For this review, take the finished solid that the model builds, in its own axes (mm). Face numbers are marked on the shaded views. A direction names the side the tool comes from. Give positions to 0.01 mm unless a question says otherwise; leave off trailing zeros. Write each loop counter-clockwise with the first axis right and the second up, starting at its lowest first coordinate (ties: lowest second). Pieces come first, ordered by that corner, then holes. Notation, with made-up numbers: M 73.25,29.25 L 80.25,29.25 A5 ccw 80.25,38.25 Z; hole C 77,60 d8. An arc over 180 degrees is marked long. Write item = value, one per line.
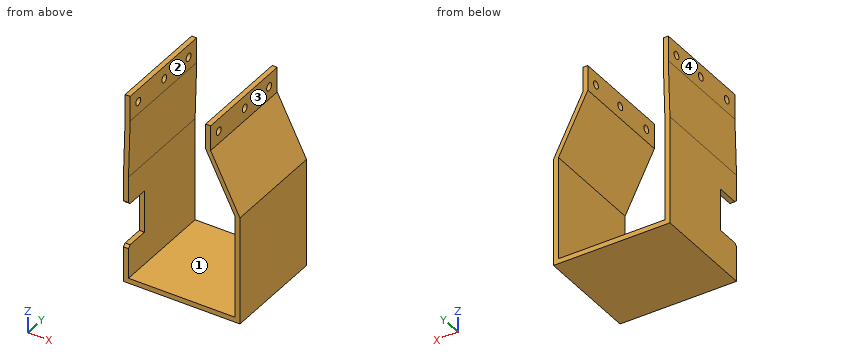
Autodesk Inventor part; units mm, degrees
ref_plane "YZ Plane" through (0, 0, 0) normal (1, 0, 0) x (0, 1, 0)
ref_plane "XZ Plane" through (0, 0, 0) normal (0, 1, 0) x (-1, 0, 0)
ref_plane "XY Plane" through (0, 0, 0) normal (0, 0, 1) x (1, 0, 0)
sketch "Sketch3" plane through (0, 0, 0) normal (0, 1, 0) x (-1, 0, 0)
  line L0 (0, 0) -> (15, 0) construction
  line L1 (0, 0) -> (-15, 0) construction
  line L2 (15, 0) -> (15, -10)
  line L3 (15, -10) -> (17, -10)
  line L4 (17, -10) -> (17, 0)
  line L5 (17, 0) -> (15, 0)
  line L6 (-15, 0) -> (-15, -10)
  line L7 (-15, -10) -> (-17, -10)
  line L8 (-17, -10) -> (-17, 0)
  line L9 (-17, 0) -> (-15, 0)
  line L10 (0, 0) -> (0, -74) construction
  line L11 (0, -74) -> (15.65, -74)
  line L12 (0, -74) -> (-26.65, -74)
  line L13 (15.65, -74) -> (15.65, -76)
  line L14 (15.65, -76) -> (-26.65, -76)
  line L15 (-26.65, -76) -> (-26.65, -74)
  line L16 (15.65, -76) -> (17.65, -76)
  line L17 (17.65, -76) -> (17.65, -33)
  line L18 (17.65, -33) -> (17, -10)
  line L19 (-26.65, -76) -> (-28.65, -76)
  line L20 (-28.65, -76) -> (-28.65, -33)
  line L21 (-28.65, -33) -> (-17, -10)
  line L22 (-26.65, -33) -> (-26.65, -74)
  line L23 (-26.65, -33) -> (-15, -10)
  line L24 (15.65, -74) -> (15.65, -33)
  line L25 (15.65, -33) -> (15, -10)
  dimension "d19" = 15
  dimension "d20" = 15
  dimension "d21" = 10
  dimension "d22" = 2
  dimension "d23" = 2
  dimension "d24" = 74
  dimension "d25" = 15.65
  dimension "d26" = 26.65
  dimension "d27" = 2
  dimension "d28" = 2
  dimension "d29" = 43
  dimension "d30" = 2
extrude "Extrusion3" add sketch "Sketch3" along normal blind 41
sketch "Sketch4" plane through (17, 0, 0) normal (1, 0, 0) x (0, 0, -1)
  line L0 (0, 41) -> (10, 41)
  line L1 (5, 41) -> (5, 0) construction
  line L2 (0, 0) -> (10, 0)
  circle A0 centre (5, 36) radius 1.5
  circle A1 centre (5, 21) radius 1.5
  circle A2 centre (5, 5) radius 1.5
  dimension "d33" = 3
  dimension "d34" = 3
  dimension "d35" = 3
  dimension "d36" = 5
  dimension "d37" = 20
  dimension "d38" = 5
extrude "Extrusion4" cut sketch "Sketch4" against normal blind 41
sketch "Sketch5" plane through (-15.65, 0, -33) normal (1, 0, 0) x (0, 0, -1)
  line L0 (43, 41) -> (0, 41) construction
  line L1 (43, 41) -> (28, 41) construction
  line L2 (28, 41) -> (11.3, 41)
  line L3 (0, 41) -> (41, 41)
  line L4 (11.3, 41) -> (11.3, 31.2)
  line L5 (11.3, 31.2) -> (28, 31.2)
  line L6 (28, 31.2) -> (28, 41)
  line L7 (-33, 0) -> (-33, 41)
  line L8 (-33, 20.5) -> (43.2926, 20.5)
  line L9 (43, 0) -> (0, 0) construction
  line L10 (28, 0) -> (11.3, 0)
  line L11 (11.3, 0) -> (11.3, 9.8)
  line L12 (11.3, 9.8) -> (28, 9.8)
  line L13 (28, 9.8) -> (28, 0)
  dimension "d41" = 15
  dimension "d42" = 16.7
  dimension "d43" = 9.8
extrude "Extrusion5" cut sketch "Sketch5" against normal blind 41 contours L10 L11 L12 L13
chamfer "Chamfer1" distance 1 angle 45 2 edges at (-16.65, 0, -61) (-16.65, 0, -44.3)
properties part number "nema 17 holder" material "Acetal Resin, Black"
1. For line 1 along Y through (x, z) = (-15.4, -5); line 2 along X through (y, z) = (5, -35.5); line 3 along Z through (x, y) = (13, 38.5), list the stretches that pass through material, from the lowest coordinate up. Write a range as from..to.
Responses:
line_1 = 0..3.5, 6.5..19.5, 22.5..34.5, 37.5..41
line_2 = -17.65..-15.65, 26.65..28.65
line_3 = -76..-74
2. We need section C-C, the plane y = 5. Write out the cut boundary in (x, z).
Responses:
outline = M -17.65,-76 L 28.65,-76 L 28.65,-33 L 17,-10 L 17,-6.5 L 15,-6.5 L 15,-10 L 26.65,-33 L 26.65,-74 L -15.65,-74 L -15.65,-61 L -17.65,-61 Z; M -17.65,-44.3 L -15.65,-44.3 L -15.65,-33 L -15,-10 L -15,-6.5 L -17,-6.5 L -17,-10 L -17.65,-33 Z; M -17,-3.5 L -15,-3.5 L -15,0 L -17,0 Z; M 15,-3.5 L 17,-3.5 L 17,0 L 15,0 Z
3. We need section B-B, the plane y = 36. Write out the cut boundary in (x, z), then the cut area to 3 significant figures.
Responses:
outline = M -17.65,-76 L 28.65,-76 L 28.65,-33 L 17,-10 L 17,-6.5 L 15,-6.5 L 15,-10 L 26.65,-33 L 26.65,-74 L -15.65,-74 L -15.65,-33 L -15,-10 L -15,-6.5 L -17,-6.5 L -17,-10 L -17.65,-33 Z; M -17,-3.5 L -15,-3.5 L -15,0 L -17,0 Z; M 15,-3.5 L 17,-3.5 L 17,0 L 15,0 Z
area = 377 mm2
4. Insertion check: P1, Ø12, axis at y = 27, z = -16.5, coming from the +X side; P2, Ø3.5, axis at y = 5, z = -5, coming from the +X side; P3, Ø5, axis at y = 20, z = -6.5, coming from the -X side. Each pin has a flat end and moves straight along its axis. Give the tip position at first contact, or say it passes through.
Responses:
P1 = 23.33
P2 = 17
P3 = -17
5. We need section D-D, the plane x = 20. Write out the cut boundary in (y, z).
Responses:
outline = M 0,-76 L 41,-76 L 41,-74 L 0,-74 Z; M 0,-19.87 L 41,-19.87 L 41,-15.92 L 0,-15.92 Z
6. We need section A-A, the plane z = -5. Count the separate pieces of the cut face and the enclosed holes in it, then the cut area to 3 significant figures.
Responses:
separate_pieces = 8
enclosed_holes = 0
area = 128 mm2
7. Machinability: for the marked faces 1, 2, 3 and 4, which of the approach directions +Z, -Z, +X, -X, +Y, -Y give a long, thin tool a straight path to every point of the face, cutting with its end or side? Answer none if there is none.
Responses:
face_1 = +Y, -Y
face_2 = +Z, +Y, -Y
face_3 = +Z, +X, +Y, -Y
face_4 = +Z, -X, +Y, -Y
